```python
from build123d import *

# Parameters (mm, degrees)
RESSALTO_EXTRUS_O1_DEPTH = 30
RESSALTO_EXTRUS_O2_DEPTH = 3
CASCA1_START             = 7
CASCA1_DEPTH             = 13
ESBO_O3_W                = 5
ESBO_O3_H                = 20
CORTE_EXTRUS_O1_DEPTH    = 67.283953563


# Read off the part's stored shape, not the designer's step: Casca1
with BuildPart() as part:
    # Esboço1 → Ressalto-extrusão1 (new body)
    with BuildSketch(Plane.XY):
        Polygon((-35, 20), (35, 20), (28.25, -21), (20.25, -21), (20.25, 0), (-20.25, 0), (-20.25, -21), (-28.25, -21), align=None)
    extrude(amount=RESSALTO_EXTRUS_O1_DEPTH)

    # Esboço2 → Ressalto-extrusão2 (add)
    with BuildSketch(Plane(origin=(0, 0, 0), x_dir=(-1, 0, 0), z_dir=(0, 0, -1))):
        Polygon((-35, 20), (35, 20), (28.25, -21), (-28.25, -21), align=None)
    extrude(amount=RESSALTO_EXTRUS_O2_DEPTH)

    # Casca1 outline → Casca1 (cut)
    with BuildSketch(Plane.XY.offset(CASCA1_START)):
        Polygon((-24.865384062, 20), (-23.219042598, 10), (23.219042598, 10), (24.865384062, 20), align=None)
    extrude(amount=CASCA1_DEPTH, mode=Mode.SUBTRACT)

    # Esboço3 → Corte-extrusão1 (cut, through all)
    with BuildSketch(Plane.ZY.offset(-20.25)):
        with Locations((7.5, -15)):
            Rectangle(ESBO_O3_W, ESBO_O3_H)
    extrude(amount=-CORTE_EXTRUS_O1_DEPTH, mode=Mode.SUBTRACT)


solid = part.part
```
Geometry: final body of the model. Coordinates: model frame, mm. A direction names the side the tool comes from. Give positions to 0.01 mm unless a question says otherwise; leave off trailing zeros. Write each loop counter-clockwise with the first axis right and the second up, starting at its lowest first coordinate (ties: lowest second). Pieces come first, ordered by that corner, then holes.
1. Reachability of faces 1 (the flat face through (24, -13, 5)), 2 (the flat face through (-24.054, 15.07, 13.409)), 3 (the flat face through (0, -10, 0)), 4 (the flat face through (0, 0, -3)) from +Z, -Z, +X, -X, +Y, -Y: full face, straight path, thin tool, end or side. Return the list, or none.
2. Section query D-D, the plane y = 13.5. Return loops of the section in (x, z).
3. Section query C-C, the plane y = -10. Return loops of the section in (x, z), then the cut area to 3 significant figures.
4. Draft query along X for faces 5 (the flat face through (0, 10, 13)), 6 (the flat face through (-21, -21, 7)), 7 (the flat face through (31.578, -0.787, 13.731)), 8 (the flat face through (0, 15, 20)). Return one class per face: released by +X, released by -X, zero draft, split by the parting line, or undercut.
5. Section query B-B, the plane z = 27.5. Return loops of the section in (x, y), then the cut area to 3 significant figures.
6. Pin query (flat end, axial travel): P1, Ø8, axis at y = 3, z = 3, coming from the -X side; P2, Ø4, axis at x = -9, z = 13, coming from the +Y side; P3, Ø2, axis at y = 4.5, z = 26, coming from the +X side; P4, Ø5.5, axis at x = 26, z = 6.5, coming from the -Y side. Return the tip coordinate at first contact, or that it passes through.
7. Line query: probe 1 along Z at (x, y) = (16, 18.5); probe 2 along Y at (x, z) = (5.5, 27.5); probe 3 along Z at (x, y) = (16, -18.5). Output: solid intervals per line, ascending.
8. Section query A-A, the plane x = 22. Return loops of the section in (y, z), then the cut area to 3 significant figures.
Computed:
1. face 1: +X, -Y
1. face 2: +Y
1. face 3: +Z, -Y
1. face 4: -Z, +X, -X, +Y, -Y
2. outline: (-33.93, -3) - (33.93, -3) - (33.93, 30) - (-33.93, 30) - close; hole (-23.8, 7) - (23.8, 7) - (23.8, 20) - (-23.8, 20) - close
3. outline: (-30.06, -3) - (30.06, -3) - (30.06, 5) - (20.25, 5) - (20.25, 0) - (-20.25, 0) - (-20.25, 30) - (-30.06, 30) - close; (20.25, 10) - (30.06, 10) - (30.06, 30) - (20.25, 30) - close
3. area: 720 mm2
4. face 5: undercut
4. face 6: zero draft
4. face 7: released by +X
4. face 8: undercut
5. outline: (-35, 20) - (-28.25, -21) - (-20.25, -21) - (-20.25, 0) - (20.25, 0) - (20.25, -21) - (28.25, -21) - (35, 20) - close
5. area: 1,740 mm2
6. P1: stops at x = -32.86
6. P2: stops at y = 10
6. P3: stops at x = 32.61
6. P4: stops at y = -21
7. probe 1: z = -3 to 7, 20 to 30
7. probe 2: y = 0 to 20
7. probe 3: z = -3 to 0
8. outline: (-21, -3) - (20, -3) - (20, 7) - (10, 7) - (10, 20) - (20, 20) - (20, 30) - (-21, 30) - (-21, 10) - (-5, 10) - (-5, 5) - (-21, 5) - close
8. area: 1,140 mm2
